Design review of the part built by this model. Coordinates are the model's own, in mm. A direction names the side the tool comes from. Give positions to 0.01 mm unless a question says otherwise; leave off trailing zeros. Loops run counter-clockwise (first coordinate to the right, second up) from the corner with the lowest first, then second, coordinate; pieces in that order, holes last. Notation, with made-up numbers: (67.5, 22) -> (88.5, 22) arc R19 ccw to (88.5, 57) -> close; hole circle Ø2 at (89.5, 74.5). An arc over 180 degrees is marked (long way). Use a Markdown table: item, result. Add a question column.
1. For pin 1 Ø12 at (y, z) = (-39, 20) entering from +X; pin 2 Ø7 at (y, z) = (-56, 4) entering from -X; pin 3 Ø5 at (x, y) = (-78.5, 39) entering from +Z, all flat-tipped, find the tip position at first contact; note any pin that passes through.
2. To check wall thickness, follow line 1 (Y direction, x = -31.75, z = 1.35); line 2 (Y direction, x = -248, z = 60); line 3 (X direction, y = -57, z = 4). State the ranges of each line that lie inside material, in increasing order.
3. Add section B-B (x = -189). State the section outline as (y, z) points.
4. For faces 5 (the flat face through (-236, 50.8, 3)), 6 (the flat face through (-261, 0, 76.2)), 7 (the flat face through (-261, 38.1, 44)), 8 (the flat face through (-158.75, 0, 3)), 9 (the flat face through (-236, -50.8, 3)), list the 3-axis set-ups (+Z, -Z, +X, -X, +Y, -Y) from which the entire face can be reached by the end or side of a thin tool; tool diameter is ignored.
5. Add section A-A (y = -57.15). State the section outline as (x, z) points.
6. Draft analysis for pull direction X (two halves, no side actions). For faces 1 (the flat face through (-99, 38.1, 3)), 2 (the flat face through (-69.85, -45, 3)), 3 (the flat face through (-285.75, -8, 78)), 4 (the flat face through (-125, 20, 0)), state which applies: pulls with the +X half, pulls with the -X half, needs draft (parallel to the pull), parting line crosses it, or undercut.
7. Add section D-D (y = 23). State the section outline as (x, z) points (3 decimals), and give its area (3 significant figures).
8. Add section C-C (z = 13.5). State the section outline as (x, y) points.
```python
from build123d import *

# Parameters (mm, degrees)
BOSS_EXTRUDE1_DEPTH       = 6.35
SKETCH5_R                 = 6.35
CUT_EXTRUDE1_DEPTH        = 202.906036314
SKETCH6_W                 = 60.96
SKETCH6_H                 = 25.4
SKETCH6_W_2               = 82.55
CUT_EXTRUDE2_DEPTH        = 10.16
M5X0_8_TAPPED_HOLE1_D     = 4.2
M5X0_8_TAPPED_HOLE1_DEPTH = 13.97
M5X0_8_TAPPED_HOLE1_TIP   = 1.2618073
SKETCH13_W                = 101.6
SKETCH13_H                = 101.6
BOSS_EXTRUDE2_DEPTH       = 6.35
SKETCH14_W                = 50.8
SKETCH14_H                = 76.2
BOSS_EXTRUDE3_DEPTH       = 76.2
SKETCH15_W                = 63.5
SKETCH15_H                = 63.5
CUT_EXTRUDE4_DEPTH        = 292.132092013
SKETCH16_W                = 25.4
SKETCH16_H                = 88.9
CUT_EXTRUDE5_DEPTH        = 3.175
SKETCH6_3_W               = 82.55
SKETCH6_3_H               = 25.4
SKETCH6_3_W_2             = 60.96
SKETCH6_3_W_3             = 69.85
CUT_EXTRUDE6_DEPTH        = 308.040722055
SKETCH17_W                = 38.1
SKETCH17_H                = 63.5
CUT_EXTRUDE7_DEPTH        = 308.040722055
SKETCH19_W                = 50.8
SKETCH19_H                = 60.96
CUT_EXTRUDE8_DEPTH        = 306.526737782
SKETCH20_W                = 50.8
SKETCH20_H                = 1.27
CUT_EXTRUDE9_DEPTH        = 306.526737782
SKETCH21_W                = 50.8
SKETCH21_H                = 1.27
CUT_EXTRUDE10_DEPTH       = 306.526737782


with BuildPart() as part:
    # Sketch2 → Boss-Extrude1 (new body)
    with BuildSketch(Plane.XY):
        Polygon((-69.85, -82.55), (-69.85, -6.35), (-19.05, -6.35), (-19.05, 82.55), (-184.15, 82.55), (-184.15, -82.55), align=None)
    extrude(amount=BOSS_EXTRUDE1_DEPTH)

    # Sketch5 → Cut-Extrude1 (cut, through all)
    with BuildSketch(Plane.XY.offset(6.35)):
        with Locations((-158.75, 57.15)):
            Circle(SKETCH5_R)
        with Locations((-158.75, -57.15)):
            Circle(SKETCH5_R)
    extrude(amount=-CUT_EXTRUDE1_DEPTH, mode=Mode.SUBTRACT)

    # Sketch6 → Cut-Extrude2 (cut)
    with BuildSketch(Plane.XY.offset(6.35)):
        with Locations((-115.57, -50.8)):
            Rectangle(SKETCH6_W, SKETCH6_H)
        with Locations((-98.425, 50.8)):
            Rectangle(SKETCH6_W_2, SKETCH6_H)
    extrude(amount=-CUT_EXTRUDE2_DEPTH, mode=Mode.SUBTRACT)

    # M5x0.8 Tapped Hole1
    with Locations(Plane.XY.offset(6.35)):
        with Locations((-31.75, 63.5), (-31.75, 38.1), (-31.75, 12.7)):
            Hole(M5X0_8_TAPPED_HOLE1_D / 2, depth=M5X0_8_TAPPED_HOLE1_DEPTH)
            with Locations((0, 0, -(M5X0_8_TAPPED_HOLE1_DEPTH + M5X0_8_TAPPED_HOLE1_TIP / 2))):  # 118° drill point
                Cone(0, M5X0_8_TAPPED_HOLE1_D / 2, M5X0_8_TAPPED_HOLE1_TIP, mode=Mode.SUBTRACT)

    # Sketch13 → Boss-Extrude2 (add)
    with BuildSketch(Plane.XY.offset(6.35)):
        with Locations((-234.95, 0)):
            Rectangle(SKETCH13_W, SKETCH13_H)
    extrude(amount=-BOSS_EXTRUDE2_DEPTH)

    # Sketch14 → Boss-Extrude3 (add)
    with BuildSketch(Plane.XY.offset(6.35)):
        with Locations((-260.35, 0)):
            Rectangle(SKETCH14_W, SKETCH14_H)
    extrude(amount=BOSS_EXTRUDE3_DEPTH)

    # Sketch15 → Cut-Extrude4 (cut, through all)
    with BuildSketch(Plane.ZY.offset(285.75)):
        with Locations((44.45, 0)):
            Rectangle(SKETCH15_W, SKETCH15_H)
    extrude(amount=-CUT_EXTRUDE4_DEPTH, mode=Mode.SUBTRACT)

    # Sketch16 → Cut-Extrude5 (cut)
    with BuildSketch(Plane.XY.offset(6.35)):
        with Locations((-31.75, 38.1)):
            Rectangle(SKETCH16_W, SKETCH16_H)
    extrude(amount=-CUT_EXTRUDE5_DEPTH, mode=Mode.SUBTRACT)

    # Sketch6_3 → Cut-Extrude6 (cut, through all)
    with BuildSketch(Plane.XY.offset(6.35)):
        with Locations((-98.425, 50.8)):
            Rectangle(SKETCH6_3_W, SKETCH6_3_H)
        with Locations((-115.57, -50.8)):
            Rectangle(SKETCH6_3_W_2, SKETCH6_3_H)
        with Locations((-123.825, 0)):
            Rectangle(SKETCH6_3_W_3, SKETCH6_3_H)
    extrude(amount=-CUT_EXTRUDE6_DEPTH, mode=Mode.SUBTRACT)

    # Sketch17 → Cut-Extrude7 (cut, through all)
    with BuildSketch(Plane.XY.offset(6.35)):
        with Locations((-203.2, 0)):
            Rectangle(SKETCH17_W, SKETCH17_H)
    extrude(amount=-CUT_EXTRUDE7_DEPTH, mode=Mode.SUBTRACT)

    # Sketch19 → Cut-Extrude8 (cut, through all)
    with BuildSketch(Plane.XY.offset(12.7)):
        with Locations((-260.35, 0)):
            Rectangle(SKETCH19_W, SKETCH19_H)
    extrude(amount=-CUT_EXTRUDE8_DEPTH, mode=Mode.SUBTRACT)

    # Sketch20 → Cut-Extrude9 (cut, through all)
    with BuildSketch(Plane.XY.offset(12.7)):
        with Locations((-260.35, 31.115)):
            Rectangle(SKETCH20_W, SKETCH20_H)
    extrude(amount=-CUT_EXTRUDE9_DEPTH, mode=Mode.SUBTRACT)

    # Sketch21 → Cut-Extrude10 (cut, through all)
    with BuildSketch(Plane.XY.offset(12.7)):
        with Locations((-260.35, -31.115)):
            Rectangle(SKETCH21_W, SKETCH21_H)
    extrude(amount=-CUT_EXTRUDE10_DEPTH, mode=Mode.SUBTRACT)


solid = part.part
```
Taken from the geometry:
| question | item | result |
|---|---|---|
| 1 | pin 1 | stops at x = -234.95 |
| 1 | pin 2 | stops at x = -184.15 |
| 1 | pin 3 | stops at z = 6.35 |
| 2 | line 1 | y = -6.35 to 10.6, 14.8 to 36, 40.2 to 61.4, 65.6 to 82.55 |
| 2 | line 2 | y = -38.1 to -31.75, 31.75 to 38.1 |
| 2 | line 3 | x = -184.15 to -165.1, -152.4 to -146.05, -85.09 to -69.85 |
| 3 | outline | (-50.8, 0) -> (-31.75, 0) -> (-31.75, 6.35) -> (-50.8, 6.35) -> close; (31.75, 0) -> (50.8, 0) -> (50.8, 6.35) -> (31.75, 6.35) -> close |
| 4 | face 5 | +Z, -Z, -X, +Y |
| 4 | face 6 | -Z, +X, -X |
| 4 | face 7 | +Z, +X, -X, +Y |
| 4 | face 8 | +Z, -Z |
| 4 | face 9 | +Z, -Z, -X, -Y |
| 5 | outline | (-184.15, 0) -> (-165.1, 0) -> (-165.1, 6.35) -> (-184.15, 6.35) -> close; (-152.4, 0) -> (-146.05, 0) -> (-146.05, 6.35) -> (-152.4, 6.35) -> close; (-85.09, 0) -> (-69.85, 0) -> (-69.85, 6.35) -> (-85.09, 6.35) -> close |
| 6 | face 1 | undercut |
| 6 | face 2 | pulls with the +X half |
| 6 | face 3 | pulls with the -X half |
| 6 | face 4 | needs draft |
| 7 | outline | (-285.75, 76.2) -> (-234.95, 76.2) -> (-234.95, 82.55) -> (-285.75, 82.55) -> close; (-234.95, 0) -> (-222.25, 0) -> (-222.25, 6.35) -> (-234.95, 6.35) -> close; (-184.15, 0) -> (-19.05, 0) -> (-19.05, 3.175) -> (-44.45, 3.175) -> (-44.45, 6.35) -> (-184.15, 6.35) -> close |
| 7 | area | 1,370 mm^2 |
| 8 | outline | (-285.75, -38.1) -> (-234.95, -38.1) -> (-234.95, -31.75) -> (-285.75, -31.75) -> close; (-285.75, 31.75) -> (-234.95, 31.75) -> (-234.95, 38.1) -> (-285.75, 38.1) -> close |
